CAD build for the part. Positions are in the model's coordinates, mm. Face numbers are marked on the shaded views. A direction names the side the tool comes from. Coordinates: 2 decimals unless noted, no trailing zeros. Loops run counter-clockwise (first coordinate to the right, second up) from the corner with the lowest first, then second, coordinate; pieces in that order, holes last. Notation, with made-up numbers: (13.25, 46.5) - (51.25, 46.5) arc R8 ccw to (51.25, 58.5) - close; hole circle Ø7 at (88.25, 49). An arc over 180 degrees is marked (long way). Put each result on its own line as item: value.
```python
from build123d import *

# Parameters (mm, degrees)
F0_W      = 152.4
F0_H      = 66.675
F1_DEPTH  = 6.35
F3_DEPTH  = 6.351
F5_DEPTH  = 6.351
F7_DEPTH  = 6.351
F9_DEPTH  = 6.351
F10_W     = 101.6
F10_H     = 66.675
F11_DEPTH = 88.9
F12_W     = 82.55
F12_H     = 53.975
F13_DEPTH = 88.9
F14_R     = 41.275
F15_DEPTH = 6.35
F17_R     = 41.275
F18_DEPTH = 6.35
F19_R     = 2.5527
F20_DEPTH = 79.376
F16_R     = 27.94
F21_DEPTH = 79.376
F22_R     = 13.97
F23_DEPTH = 12.7
F24_R     = 7.0485
F25_DEPTH = 22.2504
F26_R     = 13.97
F27_DEPTH = 12.7
F28_R     = 7.0485
F29_DEPTH = 22.2504


with BuildPart() as f1:
    # F0 (on Top) → F1 (new body)
    with BuildSketch(Plane.XY):
        with Locations((76.2, 33.3375)):
            Rectangle(F0_W, F0_H)
    extrude(amount=F1_DEPTH)

    # F2 (on face) → F3 (cut, through all)
    with BuildSketch(Plane.XY.offset(6.35)):
        with BuildLine():
            Line((146.05, 44.45), (146.05, 53.975))
            ThreePointArc((146.05, 53.975), (139.7, 60.325), (133.35, 53.975))
            Line((133.35, 53.975), (133.35, 44.45))
            Line((133.35, 44.45), (146.05, 44.45))
        make_face()
        with BuildLine():
            ThreePointArc((133.35, 44.45), (139.7, 38.1), (146.05, 44.45))
            Line((146.05, 44.45), (133.35, 44.45))
        make_face()
    extrude(amount=-F3_DEPTH, mode=Mode.SUBTRACT)

    # F4 (on face) → F5 (cut, through all)
    with BuildSketch(Plane.XY.offset(6.35)):
        with BuildLine():
            Line((133.35, 12.7), (139.7, 12.7))
            Line((139.7, 12.7), (146.05, 12.7))
            Line((146.05, 12.7), (146.05, 22.225))
            ThreePointArc((146.05, 22.225), (139.7, 28.575), (133.35, 22.225))
            Line((133.35, 22.225), (133.35, 12.7))
        make_face()
        with BuildLine():
            Line((146.05, 12.7), (139.7, 12.7))
            Line((139.7, 12.7), (133.35, 12.7))
            ThreePointArc((133.35, 12.7), (139.7, 6.35), (146.05, 12.7))
        make_face()
    extrude(amount=-F5_DEPTH, mode=Mode.SUBTRACT)

    # F6 (on face) → F7 (cut, through all)
    with BuildSketch(Plane.XY.offset(6.35)):
        with BuildLine():
            Line((6.35, 53.975), (12.7, 53.975))
            Line((12.7, 53.975), (19.05, 53.975))
            ThreePointArc((19.05, 53.975), (12.7, 60.325), (6.35, 53.975))
        make_face()
        with BuildLine():
            Line((19.05, 53.975), (12.7, 53.975))
            Line((12.7, 53.975), (6.35, 53.975))
            Line((6.35, 53.975), (6.35, 44.45))
            ThreePointArc((6.35, 44.45), (12.7, 38.1), (19.05, 44.45))
            Line((19.05, 44.45), (19.05, 53.975))
        make_face()
    extrude(amount=-F7_DEPTH, mode=Mode.SUBTRACT)

    # F8 (on face) → F9 (cut, through all)
    with BuildSketch(Plane.XY.offset(6.35)):
        with BuildLine():
            Line((6.35, 12.7), (12.7, 12.7))
            Line((12.7, 12.7), (19.05, 12.7))
            Line((19.05, 12.7), (19.05, 22.225))
            ThreePointArc((19.05, 22.225), (12.7, 28.575), (6.35, 22.225))
            Line((6.35, 22.225), (6.35, 12.7))
        make_face()
        with BuildLine():
            Line((19.05, 12.7), (12.7, 12.7))
            Line((12.7, 12.7), (6.35, 12.7))
            ThreePointArc((6.35, 12.7), (12.7, 6.35), (19.05, 12.7))
        make_face()
    extrude(amount=-F9_DEPTH, mode=Mode.SUBTRACT)

    # F10 (on face) → F11 (join)
    with BuildSketch(Plane.XY.offset(6.35)):
        with Locations((76.2, 33.3375)):
            Rectangle(F10_W, F10_H)
    extrude(amount=F11_DEPTH)

    # F12 (on face) → F13 (cut)
    with BuildSketch(Plane.XY.offset(95.25)):
        with Locations((76.2, 33.3375)):
            Rectangle(F12_W, F12_H)
    extrude(amount=-F13_DEPTH, mode=Mode.SUBTRACT)

    # F14 (on face) → F15 (join)
    with BuildSketch(Plane.XZ):
        with Locations((76.2, 47.625)):
            Circle(F14_R)
    extrude(amount=F15_DEPTH)

    # F17 (on face) → F18 (join)
    with BuildSketch(Plane(origin=(0, 66.675, 0), x_dir=(-1, 0, 0), z_dir=(0, 1, 0))):
        with Locations((-76.2, 47.625)):
            Circle(F17_R)
    extrude(amount=F18_DEPTH)

    # F19 (on face) → F20 (cut, through all)
    with BuildSketch(Plane(origin=(0, 73.025, 0), x_dir=(-1, 0, 0), z_dir=(0, 1, 0))):
        with Locations((-93.50375, 77.595974)):
            Circle(F19_R)
        with Locations((-93.50375, 17.654026)):
            Circle(F19_R)
        with Locations((-110.8075, 47.625)):
            Circle(F19_R)
        with Locations((-58.89625, 17.654026)):
            Circle(F19_R)
        with Locations((-41.5925, 47.625)):
            Circle(F19_R)
        with Locations((-58.89625, 77.595974)):
            Circle(F19_R)
    extrude(amount=-F20_DEPTH, mode=Mode.SUBTRACT)

    # F16 (on face) → F21 (cut, through all)
    with BuildSketch(Plane.XZ.offset(6.35)):
        with Locations((76.2, 47.625)):
            Circle(F16_R)
    extrude(amount=-F21_DEPTH, mode=Mode.SUBTRACT)

    # F22 (on face) → F23 (join)
    with BuildSketch(Plane(origin=(25.4, 0, 0), x_dir=(0, -1, 0), z_dir=(-1, 0, 0))):
        with Locations((-33.3375, 74.93)):
            Circle(F22_R)
    extrude(amount=F23_DEPTH)

    # F24 (on face) → F25 (cut)
    with BuildSketch(Plane(origin=(12.7, 0, 0), x_dir=(0, -1, 0), z_dir=(-1, 0, 0))):
        with Locations((-33.3375, 74.93)):
            Circle(F24_R)
    extrude(amount=-F25_DEPTH, mode=Mode.SUBTRACT)

    # F26 (on face) → F27 (join)
    with BuildSketch(Plane.YZ.offset(127)):
        with Locations((33.3375, 74.93)):
            Circle(F26_R)
    extrude(amount=F27_DEPTH)

    # F28 (on face) → F29 (cut)
    with BuildSketch(Plane.YZ.offset(139.7)):
        with Locations((33.3375, 74.93)):
            Circle(F28_R)
    extrude(amount=-F29_DEPTH, mode=Mode.SUBTRACT)


solid = f1.part
```
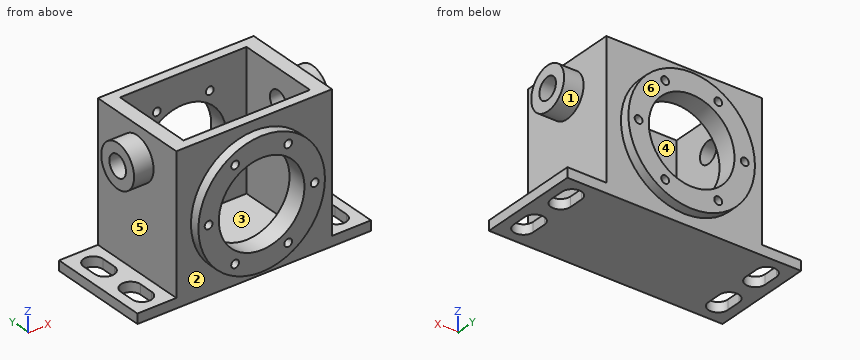
Q1. Wall check: L1, parallel to Y at x = 101, z = 61 (3 decimals); L2, parallel to X at y = 14, z = 44 (3 decimals). Give the ranges that are in metal, low to high. Write a range as from..to.
Determined:
L1: -6.35..6.35, 60.325..73.025
L2: 25.4..34.925, 117.475..127
Q2. Tool access for the marked faces 1, 2 and 3: list every direction of +Z, -Z, +X, -X, +Y, -Y with a clear straight run to the whole face (end or side of a thin tool).
Determined:
face 1: +X
face 2: -Y
face 3: +Z
Q3. Pin check, flat tips, straight feed: pin 1 Ø8.5 at (y, z) = (33.34, 74.93) entering from -X; pin 2 Ø5 at (y, z) = (19, 20.5) entering from +X; pin 3 Ø1 at (x, z) = (41.5, 17.5) entering from +Y (3 decimals); pin 4 Ø16 at (y, z) = (31, 50) entering from -X. Stop position of each tip, or through.
Determined:
pin 1: through
pin 2: x = 127
pin 3: y = 66.675
pin 4: x = 25.4
Q4. Slice it at A-A, the plane x = 77. Give the cut face in (y, z) (3 decimals), then the cut area to 3 significant figures.
Determined:
outline: (-6.35, 6.358) - (0, 6.358) - (0, 0) - (66.675, 0) - (66.675, 6.358) - (73.025, 6.358) - (73.025, 19.696) - (60.325, 19.696) - (60.325, 6.35) - (6.35, 6.35) - (6.35, 19.696) - (-6.35, 19.696) - close; (-6.35, 75.554) - (6.35, 75.554) - (6.35, 95.25) - (0, 95.25) - (0, 88.892) - (-6.35, 88.892) - close; (60.325, 75.554) - (73.025, 75.554) - (73.025, 88.892) - (66.675, 88.892) - (66.675, 95.25) - (60.325, 95.25) - close
area: 1,180 mm2
Q5. Slice it at C-C, the plane y = 63. State how many separate pieces and enclosed holes the cut face has, then the cut area to 3 significant figures.
Determined:
separate pieces: 1
enclosed holes: 7
area: 7,420 mm2
Q6. Slice it at B-B, the plane z = 38.5. Give the cut face in (x, y) (3 decimals).
Determined:
outline: (25.4, 0) - (35.946, 0) - (35.946, -6.35) - (49.792, -6.35) - (49.792, 6.35) - (34.925, 6.35) - (34.925, 60.325) - (49.792, 60.325) - (49.792, 73.025) - (35.946, 73.025) - (35.946, 66.675) - (25.4, 66.675) - close; (102.608, -6.35) - (116.454, -6.35) - (116.454, 0) - (127, 0) - (127, 66.675) - (116.454, 66.675) - (116.454, 73.025) - (102.608, 73.025) - (102.608, 60.325) - (117.475, 60.325) - (117.475, 6.35) - (102.608, 6.35) - close
Q7. Mould opens along X. For the marked faces 4, 5 and 6 say: +X half, -X half, draft (parallel to the pull), parting line (faces both ways), or undercut.
Determined:
face 4: undercut
face 5: -X half
face 6: draft
Q8. Slice it at D-D, the plane y = 42. Give the cut face in (x, z) (3 decimals), then the cut area to 3 significant figures.
Determined:
outline: (0, 0) - (6.842, 0) - (6.842, 6.35) - (0, 6.35) - close; (12.7, 63.97) - (25.4, 63.97) - (25.4, 6.35) - (18.558, 6.35) - (18.558, 0) - (133.842, 0) - (133.842, 6.35) - (127, 6.35) - (127, 63.97) - (139.7, 63.97) - (139.7, 85.89) - (127, 85.89) - (127, 95.25) - (117.475, 95.25) - (117.475, 6.35) - (34.925, 6.35) - (34.925, 95.25) - (25.4, 95.25) - (25.4, 85.89) - (12.7, 85.89) - close; (145.558, 0) - (152.4, 0) - (152.4, 6.35) - (145.558, 6.35) - close
area: 3,070 mm2
